from build123d import *

# Parameters (mm, degrees)
F1_DEPTH = 18
F5_R     = 0.2


with BuildPart() as f1:
    # F0 (on Right) → F1 (new body)
    with BuildSketch(Plane.YZ):
        Polygon((-32.2547115611, 1.6), (-32.2547115611, 0), (-27.3547115611, 0), (-25.7547115611, 1.6), (-25.7547115611, 1.8), (-25.9547115611, 1.8), (-26.886082411, 2.7313708499), (-28.0174532609, 1.6), (-31.2547115611, 1.6), (-31.2547115611, 1.7), (-32.2547115611, 1.7), align=None)
    extrude(amount=F1_DEPTH)

    # F4: F1 across plane


with BuildPart() as f1_1:
    add(f1.part)
    add(f1.part.mirror(Plane.XZ.offset(25.7547115611)))

    # F5
    f5_edges = [f1_1.edges().sort_by_distance(p)[0] for p in [
        (9, -25.554712, 1.8),
        (9, -25.954712, 1.8),
        (9, -25.754712, 1.6),
        (9, -24.623341, 2.731371),
        (9, -26.886082, 2.731371),
    ]]
    fillet(f5_edges, radius=F5_R)


solid = f1_1.part
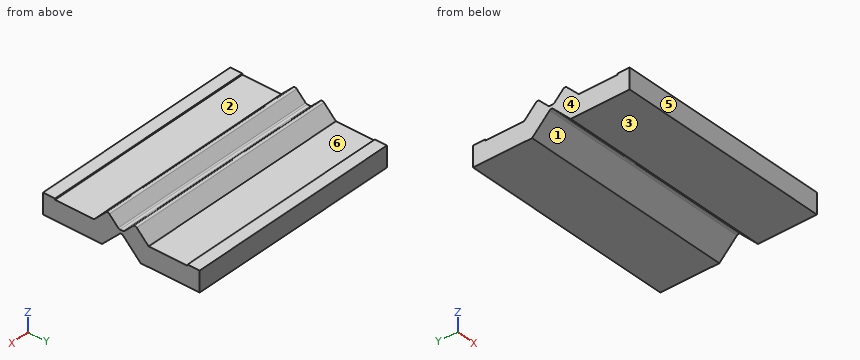
CAD build for the part. Positions are in the model's coordinates, mm. Face numbers are marked on the shaded views. A direction names the side the tool comes from. Coordinates: 2 decimals unless noted, no trailing zeros. Loops run counter-clockwise (first coordinate to the right, second up) from the corner with the lowest first, then second, coordinate; pieces in that order, holes last. Notation, with made-up numbers: (70.5, 55) - (81.5, 55) arc R14 cw to (81.5, 71) - close; hole circle Ø6 at (28, -40). An arc over 180 degrees is marked (long way). Use one line per item in the form item = value. Start each with the question number.
1) Drill centre lines: L1, parallel to Z at x = 9, y = -29.75; L2, parallel to Y at x = 6, z = 2; L3, parallel to Y at x = 4, z = 0.35. Where is each one in solid material? Low to high. Write a range as from..to.
2) Band-saw the part on D-D (z = 1.2). Give the cut face in (x, y), and give its area (3 significant figures).
3) Band-saw the part on A-A (z = 0.4). Give the cut face in (x, y), and give its area (3 significant figures).
4) Flat gauge pins, fed straight in: pin 1 (1 mm diameter, centred on x = 8.5, z = 2.5, fed in from +Y); pin 2 (1.1 mm diameter, centred on x = 13, y = -32, fed in from +Z); pin 3 (3.5 mm diameter, centred on x = 8.5, y = -22.5, fed in from +Z); pin 4 (2 mm diameter, centred on x = 4.5, y = -20.5, fed in from -Z). Where does each tip first touch, or does it go through?
5) Band-saw the part on B-B (x = 3.5). Give the cut face in (y, z).
6) Tool access for the marked faces 1, 2 and 3: list every direction of +Z, -Z, +X, -X, +Y, -Y with a clear straight run to the whole face (end or side of a thin tool).
7) Two-plate mould, pull along Y, no slides. Class the marked faces 4, 5 and 6: +Y half, -Y half, draft (parallel to the pull), parting line (faces both ways), or undercut.
8) Band-saw the part on C-C (y = -22). Give the cut face in (x, z).
Check values:
q1.L1 = 0..1.6
q1.L2 = -27.62..-26.15, -25.35..-23.89
q1.L3 = -32.25..-27, -24.5..-19.25
q2.outline = (0, -32.25) - (18, -32.25) - (18, -26.15) - (0, -26.15) - close; (0, -25.35) - (18, -25.35) - (18, -19.25) - (0, -19.25) - close
q2.area = 220 mm2
q3.outline = (0, -32.25) - (18, -32.25) - (18, -26.95) - (0, -26.95) - close; (0, -24.55) - (18, -24.55) - (18, -19.25) - (0, -19.25) - close
q3.area = 191 mm2
q4.pin_1 = -23.89
q4.pin_2 = 1.7
q4.pin_3 = 2.36
q4.pin_4 = 0
q5.outline = (-32.25, 0) - (-27.35, 0) - (-25.9, 1.46) arc R0.2 cw to (-25.61, 1.46) - (-24.15, 0) - (-19.25, 0) - (-19.25, 1.7) - (-20.25, 1.7) - (-20.25, 1.6) - (-23.49, 1.6) - (-24.48, 2.59) arc R0.2 ccw to (-24.76, 2.59) - (-25.5, 1.86) arc R0.2 cw to (-25.64, 1.8) - (-25.87, 1.8) arc R0.2 cw to (-26.01, 1.86) - (-26.74, 2.59) arc R0.2 ccw to (-27.03, 2.59) - (-28.02, 1.6) - (-31.25, 1.6) - (-31.25, 1.7) - (-32.25, 1.7) - close
q6.face_1 = -Z, +X, -X
q6.face_2 = +Z, +X, -X
q6.face_3 = -Z, +X, -X, +Y, -Y
q7.face_4 = draft
q7.face_5 = -Y half
q7.face_6 = undercut
q8.outline = (0, 0) - (18, 0) - (18, 1.6) - (0, 1.6) - close
